Source: CAD feature listing. Evaluate the final solid. Frame: model axes, mm. A direction names the side the tool comes from. Give positions to 0.01 mm unless a question says otherwise; leave off trailing zeros. Loops run counter-clockwise (first coordinate to the right, second up) from the corner with the lowest first, then second, coordinate; pieces in that order, holes last. Notation, with made-up numbers: M 33.5,-30.5 L 65.5,-30.5 A32 cw 65.5,-2.5 Z; hole C -34.5,56.5 d9. An arc over 180 degrees is marked long. Write item = value, one per line.
from build123d import *

# Parameters (mm, degrees)
F0_W        = 95.0020104647
F0_H        = 107.3112413287
F1_DEPTH    = 254
F2_T1_DEPTH = 655.5528673222
F3_W        = 69.5454850793
F3_H        = 60.9275996685


# Not quite as in the source:
# - a fillet or chamfer that OpenCascade refuses, or shapes differently, is made with other operations: its cross-section is extruded or revolved along the edge and cut away or added


with BuildPart() as f1:
    # F0 (on Top) → F1 (new body)
    with BuildSketch(Plane.XY):
        Rectangle(F0_W, F0_H)
    extrude(amount=F1_DEPTH)

    # F2: fillet of radius 112.2174748062 on 1 edges, made by hand

    # F2_s2 → F2_t1 (cut)
    with BuildSketch(Plane.YZ.offset(-327.7764336611)):
        with BuildLine():
            ThreePointArc((53.6556206644, 141.8898286285), (22.5039425406, 219.4855647234), (-53.6556206644, 254))
            Line((-53.6556206644, 254), (53.6556206644, 254))
            Line((53.6556206644, 254), (53.6556206644, 141.8898286285))
        make_face()
    extrude(amount=F2_T1_DEPTH, mode=Mode.SUBTRACT)

    # F4: sweep along a path in F4_path
    with BuildLine(Plane(origin=(-47.5010052323, -53.6556206644, 254), x_dir=(0, 0, 1), z_dir=(1, 0, 0))) as f4_path:
        ThreePointArc((0, 0), (-34.5144352766, -76.159563205), (-112.1101713715, -107.3112413288))
        Line((-112.1101713715, -107.3112413288), (-254, -107.3112413288))
    # F3 (on face) → F4 (sweep, cut)
    with BuildSketch(Plane.XZ.offset(53.6556206644)):
        with Locations((0, 208.4547877312)):
            Rectangle(F3_W, F3_H)
    sweep(path=f4_path.line, mode=Mode.SUBTRACT)


solid = f1.part
1. Pull-direction query (Z, two-part tool) for faces 1 (the flat face through (34.773, 4, 118)), 2 (the flat face through (47.501, -1, 125)), 3 (the cylindrical face through (-0.5, 11.4, 209.3)), 4 (the flat face through (-1, -23, 0)); classes: +Z half, -Z half, draft (parallel to the pull), parting line (faces both ways), or undercut.
Derived:
face_1 = undercut
face_2 = draft
face_3 = undercut
face_4 = -Z half
2. Cut plane B-B, the plane x = -23.5. Return the cut outline in (y, z), then the cut area to 3 significant figures.
Derived:
outline = M -53.66,0 L -22.28,0 L -22.28,138.57 A36.43 ccw -53.66,177.99 Z; M -53.66,238.92 A97.15 cw 38.59,141.23 L 38.59,0 L 53.66,0 L 53.66,141.89 A112.22 ccw -53.66,254 Z
area = 9,860 mm²
3. Material intervals for probe 1 along X at (y, z) = (-36, 226); probe 2 along Y at (x, z) = (3, 51); probe 3 along Z at (x, y) = (32, -28.5), sorted ascending. Write a range as from..to.
Derived:
probe_1 = -47.5..-34.77, 34.77..47.5
probe_2 = -53.66..-22.28, 38.59..53.66
probe_3 = 0..162.47, 234.27..250.01
4. Cut plane D-D, the plane z = 218. Return the cut outline in (x, y), then the cut area to 3 significant figures.
Derived:
outline = M -47.5,-53.66 L -34.77,-53.66 L -34.77,1.82 L 34.77,1.82 L 34.77,-53.66 L 47.5,-53.66 L 47.5,23.9 L -47.5,23.9 Z
area = 3,510 mm²
5. Reachability of faces 5 (the cylindrical face through (-0.665, 23.329, 218.615)), 6 (the flat face through (0, 38.589, 70)), 7 (the flat face through (-34.773, 5, 118)) from +Z, -Z, +X, -X, +Y, -Y: full face, straight path, thin tool, end or side. Return the list, or none.
Derived:
face_5 = +Z, +X, -X, +Y
face_6 = -Z
face_7 = none
6. Cut plane C-C, the plane y = -31.5. Return the cut outline in (x, z), then the cut area to 3 significant figures.
Derived:
outline = M -47.5,0 L 47.5,0 L 47.5,250.8 L -47.5,250.8 Z; hole M -34.77,166.28 L 34.77,166.28 L 34.77,235.2 L -34.77,235.2 Z
area = 19,000 mm²
7. First-contact query: pin 1 Ø8 at (x, y) = (-15, -39.5) entering from -Z; pin 2 Ø2 at (x, z) = (-31.5, 193.5) entering from +Y. Flat tips, straight axial feed; report the tip coordinate or a pass-through.
Derived:
pin_1 = 0
pin_2 = 41.59
8. Cut plane A-A, the plane z = 78. Return the cut outline in (x, y).
Derived:
outline = M -47.5,-53.66 L 47.5,-53.66 L 47.5,53.66 L -47.5,53.66 Z; hole M -34.77,-22.28 L 34.77,-22.28 L 34.77,38.59 L -34.77,38.59 Z
